Geometry: final body of the model. Coordinates: model frame, mm. A direction names the side the tool comes from. Round coordinates to 2 decimals unless told otherwise and drop trailing zeros. Write each loop counter-clockwise with the first axis right and the second up, starting at its lowest first coordinate (ties: lowest second). Pieces come first, ordered by that corner, then holes. Notation, with made-up numbers: (-31.75, -31.75) - (-7.75, -31.75) arc R23 cw to (-7.75, -11.75) - close; hole circle Ø3 at (77, 10.25). An arc over 180 degrees is marked (long way). Use a Markdown table: item, result. Add a question column.
```python
from build123d import *

# Parameters (mm, degrees)
BASPROSKE_W                  = 5
BASPROSKE_H                  = 13.5
TOOTHCUT_DEPTH               = 20.735754356
TEETHCUTS_COUNT              = 25
TEETHCUTS_ANGLE              = 345.6
BORSKE_R                     = 4.5
BORE_DEPTH                   = 50.0000508
ESQUISSE3_R                  = 2.1
ENL_V_MAT_EXTRU_1_DEPTH      = 20.727564352
R_P_TITION_CIRCULAIRE1_COUNT = 2


with BuildPart() as part:
    # BasProSke → Base-Revolve (revolve)
    with BuildSketch(Plane(origin=(0, 0, 0), x_dir=(1, 0, 0), z_dir=(0, 1, 0)), mode=Mode.PRIVATE) as base_revolve_sk:
        with Locations((2.5, 6.75)):
            Rectangle(BASPROSKE_W, BASPROSKE_H)
    revolve(base_revolve_sk.sketch.rotate(Axis((-10, 0, 0), (1, 0, 0)), 180), axis=Axis((-10, 0, 0), (1, 0, 0)))

    # TooCutSke → ToothCut (cut, through all)
    with BuildSketch(Plane(origin=(0, 0, 0), x_dir=(0, 0, -1), z_dir=(1, 0, 0))):
        with BuildLine():
            ThreePointArc((0.480087995, 11.238750665), (0, 11.249), (-0.480087995, 11.238750665))
            ThreePointArc((-0.480087995, 11.238750665), (-0.821124963, 12.40220054), (-1.432168974, 13.449361962))
            ThreePointArc((-1.432168974, 13.449361962), (0, 13.5254), (1.432168974, 13.449361962))
            ThreePointArc((1.432168974, 13.449361962), (0.821124963, 12.40220054), (0.480087995, 11.238750665))
        make_face()
    toothcut = extrude(amount=TOOTHCUT_DEPTH, mode=Mode.SUBTRACT)

    # TeethCuts: ToothCut ×25 about axis
    teethcuts_axis = Axis((-10, 0, 0), (1, 0, 0))
    for i in range(1, TEETHCUTS_COUNT):
        add(toothcut.rotate(teethcuts_axis, i * TEETHCUTS_ANGLE / (TEETHCUTS_COUNT - 1)), mode=Mode.SUBTRACT)

    # BorSke → Bore (cut, symmetric)
    with BuildSketch(Plane(origin=(0, 0, 0), x_dir=(0, 0, -1), z_dir=(1, 0, 0))):
        with Locations(Location((0, 0, 0), (0, 0, 180))):
            Circle(BORSKE_R)
    extrude(amount=BORE_DEPTH, both=True, mode=Mode.SUBTRACT)

    # Esquisse3 → Enlèv. mat.-Extru.1 (cut, through all)
    with BuildSketch(Plane.ZY):
        with Locations((-2.072553705, 7.78)):
            Circle(ESQUISSE3_R)
    enl_v_mat_extru_1 = extrude(amount=-ENL_V_MAT_EXTRU_1_DEPTH, mode=Mode.SUBTRACT)

    # Répétition circulaire1: Enlèv. mat.-Extru.1 ×2 about axis
    r_p_tition_circulaire1_axis = Axis((0, 0, 0), (1, 0, 0))
    for i in range(1, R_P_TITION_CIRCULAIRE1_COUNT):
        add(enl_v_mat_extru_1.rotate(r_p_tition_circulaire1_axis, i * 360 / R_P_TITION_CIRCULAIRE1_COUNT), mode=Mode.SUBTRACT)


solid = part.part
```
1) Section C-C, the plane y = -3.25. Return the cut outline in (x, z).
2) Pin query (flat end, axial travel): P1, Ø3, axis at x = 3.5, z = -8.5, coming from the +Y side; P2, Ø1.5, axis at x = 4.5, z = 4.5, coming from the +Y side; P3, Ø2, axis at x = 2, y = -4.5, coming from the +Z side; P4, Ø5.5, axis at y = 0, z = 0, coming from the -X side. Return the tip coordinate at first contact, or that it passes through.
3) Section A-A, the plane y = -6.25. Return the cut outline in (x, z).
4) Section B-B, the plane x = 2. State how many separate pieces and enclosed holes the cut face has, then the cut area to 3 significant figures.
5) Draft query along Y for faces 1 (the cylindrical face through (2.46, 11.25, -0.01)), 2 (the cylindrical face through (2.465, 5.947, 10.88)), 3 (the cylindrical face through (2.46, -11.16, -1.4)), 4 (the flat face through (0, -6, 0)). Return one class per face: released by +Y, released by -Y, zero draft, split by the parting line, or undercut.
6) Set-up query: faces 5 (the cylindrical face through (2.465, 0.713, 11.226)), 6 (the cylindrical face through (2.46, 12.4, -0.82)), 7 (the cylindrical face through (2.46, -11.16, 1.42)), 8 (the cylindrical face through (2.465, 3.054, 12.017)). Return all of +Z, -Z, +X, -X, +Y, -Y with unobstructed straight access to the full face (end or side cutting, diameter ignored); none if empty.
7) Material intervals for L1, parallel to Y at x = 0.65, z = -1.75; L2, parallel to Y at x = 3.35, z = -2.75; L3, parallel to Z at x = 4.85, y = -7, sorted ascending. Write a range as from..to.
Output values:
| question | item | result |
|---|---|---|
| 1 | outline | (0, -12.2) - (5, -12.2) - (5, -3.11) - (0, -3.11) - close; (0, 3.11) - (5, 3.11) - (5, 12.2) - (0, 12.2) - close |
| 2 | P1 | stops at y = 11.08 |
| 2 | P2 | stops at y = 12.65 |
| 2 | P3 | stops at z = 12.92 |
| 2 | P4 | passes through |
| 3 | outline | (0, -11.06) - (5, -11.06) - (5, 0.63) - (0, 0.63) - close; (0, 3.51) - (5, 3.51) - (5, 11.06) - (0, 11.06) - close |
| 4 | separate pieces | 1 |
| 4 | enclosed holes | 3 |
| 4 | area | 386 mm^2 |
| 5 | face 1 | released by +Y |
| 5 | face 2 | undercut |
| 5 | face 3 | released by -Y |
| 5 | face 4 | zero draft |
| 6 | face 5 | +Z, +X, -X |
| 6 | face 6 | +X, -X, +Y |
| 6 | face 7 | +X, -X, -Y |
| 6 | face 8 | +X, -X |
| 7 | L1 | y = -11.11..-4.15, 4.15..5.7, 9.86..13.39 |
| 7 | L2 | y = -12.76..-3.56, 3.56..5.79, 9.77..10.91 |
| 7 | L3 | z = -11.54..-9.36, -8.81..0.12, 4.02..8.81, 9.36..11.54 |
